The listing builds one solid part. Answer for the finished solid, in the listing's coordinates (mm). A direction names the side the tool comes from. Give positions to 0.01 mm unless a question says otherwise; leave off trailing zeros. Loops run counter-clockwise (first coordinate to the right, second up) from the corner with the lowest first, then second, coordinate; pieces in that order, holes last. Notation, with made-up numbers: M -11,0.5 L 14,0.5 A32 ccw 14,34.5 Z; hole C 29.25,-27 d8. An arc over 180 degrees is marked long. Return JSON: item names as keys, results as strings.
from build123d import *

# Parameters (mm, degrees)
F0_R     = 11.43
F1_DEPTH = 19.05
F4_DEPTH = 2.032
F5_DEPTH = 2.032
F7_DEPTH = 2.04216
F9_DEPTH = 2.032


# Not quite as in the source:
# - the program builds the solid bodies; features that only make, move or delete a surface that nothing else refers to are left out


with BuildPart() as f1:
    # F0 (on Top) → F1 (new body)
    with BuildSketch(Plane.XY):
        Circle(F0_R)
    extrude(amount=F1_DEPTH)

    # F2 (on face) → F4 (join)
    with BuildSketch(Plane.XY.offset(19.05)):
        Polygon((-1.880699303, -9.8758544773), (-1.880699303, -9.2042507604), (-1.9244262949, -9.0331919491), (-1.9849389791, -8.9233731851), (-2.1037228871, -8.7844179943), (-2.2359541617, -8.6320163682), (-2.3368084803, -8.5490914062), (-2.4040446151, -8.5124997422), (-4.8866966505, -8.5124997422), (-4.8866966505, -10.3327196733), (-1.880699303, -10.3327196733), align=None)
    extrude(amount=F4_DEPTH)

    # F3 (on face) → F5 (join)
    with BuildSketch(Plane.XY.offset(19.05)):
        Polygon((-1.7278705491, -8.1480639055), (-1.2155624572, -8.848301135), (-0.99472492, -9.0333931148), (-0.6215886096, -9.2146312818), (-0.2580773879, -9.3326671917), (0.2562761689, -9.4326803476), (-2.7548340149, -0.7004765794), (2.3825464305, -0.7004765794), (2.8303356376, -0.6551945116), (3.0876482706, -0.5188287272), (3.3525165636, -0.1815205032), (3.8505939301, 1.2300182134), (4.0490847188, 2.823865274), (4.0490847188, 3.8342506159), (4.0490847188, 4.6603621612), (3.7003470565, 5.6716995562), (3.3525165636, 6.6804061644), (2.7548240032, 7.6480992138), (2.1429003682, 8.4734838456), (1.3896959743, 9.2225758454), (0.4744292394, 9.9412809361), (0.1303268877, 10.2114842576), (-0.2051776682, 10.0957928225), (-0.6890241057, 9.7257923335), (-1.3436399167, 9.1707920656), (-1.9814397674, 8.4734838456), (-2.7524866164, 7.4915601872), (-3.3928717021, 6.4100213349), (-4.0235333078, 4.9190376551), (-4.2040259577, 3.9907894097), (-4.4032568112, 2.966173226), (-4.5597953722, 1.3723261654), (-4.5597953722, 0.5327102263), (-4.5597953722, -0.4492135195), (-4.5597953722, -1.1038292432), (-4.4032568112, -1.8722912064), (-4.1837464389, -2.9998348066), (-3.9051796775, -3.8076769561), (-3.6632562988, -4.519215785), (-3.5209483467, -4.9319081008), (-3.0940251891, -5.8569088578), (-2.6955632493, -6.5826787613), (-2.1829206962, -7.4222944677), align=None)
    extrude(amount=F5_DEPTH)

    # F6 (on face) → F7 (cut)
    with BuildSketch(Plane.XY.offset(21.082)):
        Polygon((1.3896959743, 9.2225758454), (-2.7548340149, -0.7004765794), (2.3825464305, -0.7004765794), (2.8303356376, -0.6551945116), (3.0876482706, -0.5188287272), (3.3525165636, -0.1815205032), (3.8505939301, 1.2300182134), (4.0490847188, 2.823865274), (4.0490847188, 4.6603621612), (3.3525165636, 6.6804061644), (2.7548240032, 7.6480992138), (2.1429003682, 8.4734838456), align=None)
    extrude(amount=-F7_DEPTH, mode=Mode.SUBTRACT)

    # F8 (on face) → F9 (join)
    with BuildSketch(Plane.XY.offset(19.03984)):
        Polygon((1.94505778, 8.4734838456), (1.3896959743, 9.2225758454), (-0.0989583414, 5.6583611201), (2.5561635848, 4.8432974145), (2.6805696543, 5.3959228098), (2.7548240032, 5.8293724433), (2.7548240032, 6.2017086893), (2.5935345329, 7.0562646724), (2.3686850909, 7.748354692), align=None)
    extrude(amount=F9_DEPTH)


solid = f1.part
(1) The part is cut by section A-A (z = 16.5). Determine the outline of the cut face in (x, y).
Values follow:
{"outline": "C 0,0 d22.86"}
(2) A tool of negligible diameter and unlimited length cuts with its end or side. For faces 4 (the flat face through (-1.881, -10, 20)), 5 (the flat face through (2.675, 6.623, 20.042)), 6 (the flat face through (-4.48, 2.18, 20.05)), 7 (the flat face through (-4.3, -2.4, 20.1)), from which of +Z, -Z, +X, -X, +Y, -Y can it reach the whole face along a straight path? Write none if from no direction.
Values follow:
{"face 4": "+Z, -Y", "face 5": "+Z, +X, +Y", "face 6": "+Z, -X, +Y", "face 7": "+Z, -X"}
(3) The part is cut by section B-B (x = -5.5). Determine the outline of the cut face in (y, z).
Values follow:
{"outline": "M -10.02,0 L 10.02,0 L 10.02,19.05 L -10.02,19.05 Z"}
(4) The part is cut by section C-C (x = 8.5). Determine the outline of the cut face in (y, z).
Values follow:
{"outline": "M -7.64,0 L 7.64,0 L 7.64,19.05 L -7.64,19.05 Z"}
(5) Determine the mould class of faces 1 (the flat face through (1.21, 5.257, 20.042)), 2 (the flat face through (-2, 3, 21.082)), 3 (the flat face through (-3.31, -5.39, 20.05)) for opening direction X: released by +X, released by -X, zero draft, split by the parting line, or undercut.
Values follow:
{"face 1": "undercut", "face 2": "zero draft", "face 3": "released by -X"}
(6) Straight lines are drawn through the part: line 1 along Z through (x, y) = (4, -5.25); line 2 along Y through (x, z) = (4.75, 3.25); line 3 along X through (y, z) = (3.5, 12.5). For each, find the intervals that lie inside material, in ascending order.
Values follow:
{"line 1": "0 to 19.05", "line 2": "-10.4 to 10.4", "line 3": "-10.88 to 10.88"}
(7) Given pin 1 (0.9 mm diameter, centred on x = 1.5, y = 6.5, fed in from +Z); pin 2 (1.6 mm diameter, centred on y = 0, z = 20, fed in from -X); pin 3 (4 mm diameter, centred on y = 6.5, z = 11.5, fed in from +X), each flat-ended and moving along its own axis, determine where each tip first touches the part or whether it passes through.
Values follow:
{"pin 1": "z = 21.07", "pin 2": "x = -4.56", "pin 3": "x = 10.51"}
